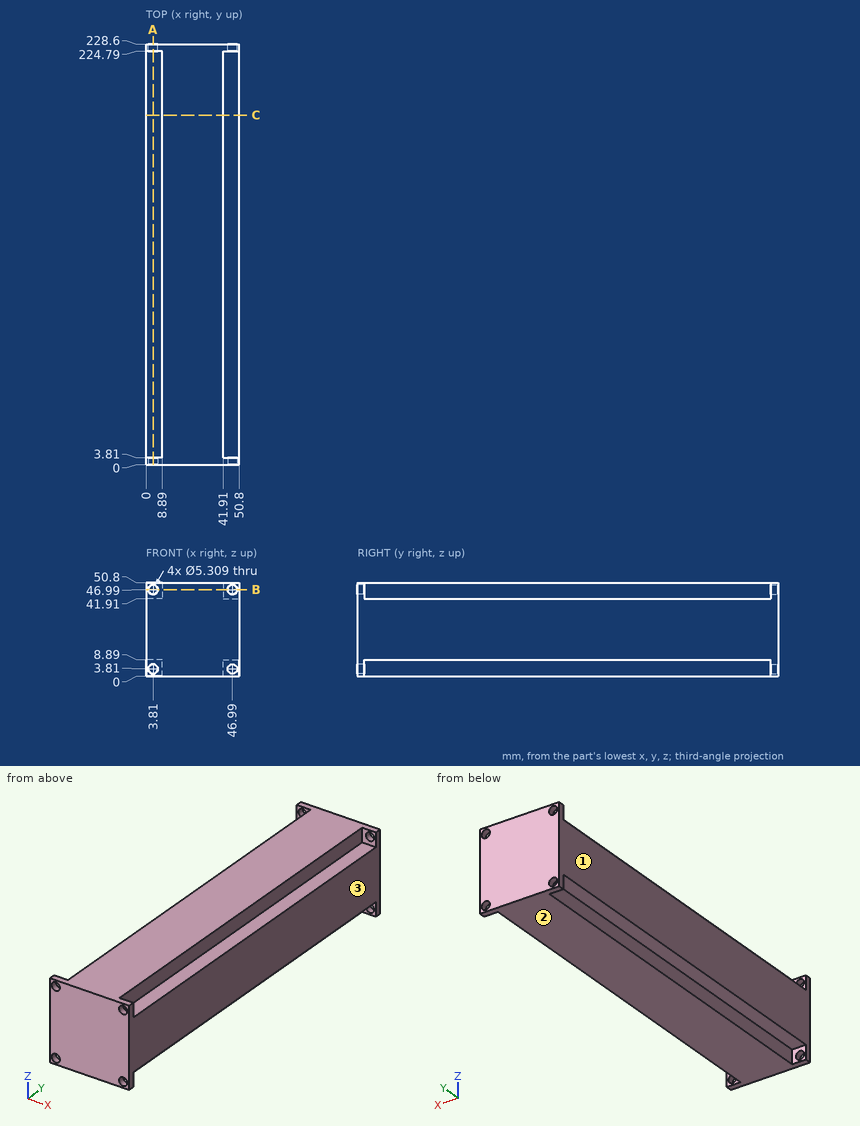
For this review, use the dimensioned drawing (mm, ordinates from the lowest corner) and the shaded views. Give positions to 0.01 mm unless a question says otherwise; leave off trailing zeros. Write each loop counter-clockwise with the first axis right and the second up, starting at its lowest first coordinate (ties: lowest second). Pieces come first, ordered by that corner, then holes. Notation, with made-up numbers: M 10.5,-26 L 36.5,-26 A21 ccw 36.5,8 Z; hole C 89.25,14 d7. An arc over 180 degrees is marked long. Answer as a JSON object with one key per item and string values. Group by question number.
1) For line 1 along Z through (x, y) = (3.81, 1.15) (1 decimal); line 2 along Z through (x, y) = (46, 1), list the stretches that pass through material, from the lowest coordinate up.
2) We need section A-A (x = 3.81). Give the boundary of the cut face in (y, z) (1 decimal).
3) Clearance check with flat-ended pins moving along their axes: pin 1 Ø7 at (x, z) = (47.5, 4.5) entering from -Y; pin 2 Ø4.5 at (y, z) = (122.5, 47.5) entering from +X; pin 3 Ø10 at (y, z) = (95.5, 47.5) entering from -X. State where each tip first meets the part, or that it passes through.
4) We need section C-C (y = 190). Give the boundary of the cut face in (x, z), and give its area (3 significant figures).
5) Mouldability with a two-part tool opening along X and no side actions: class the marked faces 1, 2 and 3 as released by +X, released by -X, zero draft, split by the parting line, or undercut.
6) We need section B-B (z = 46.99). Give the boundary of the cut face in (x, y) (1 decimal).
Answer key:
{
 "1": {"line 1": "z = 0 to 1.2, 6.5 to 44.3, 49.6 to 50.8", "line 2": "z = 0 to 1.35, 6.27 to 44.53, 49.45 to 50.8"},
 "2": {"outline": "M 0,0 L 3.8,0 L 3.8,1.2 L 0,1.2 Z; M 0,6.5 L 3.8,6.5 L 3.8,8.9 L 224.8,8.9 L 224.8,6.5 L 228.6,6.5 L 228.6,44.3 L 224.8,44.3 L 224.8,41.9 L 3.8,41.9 L 3.8,44.3 L 0,44.3 Z; M 0,49.6 L 3.8,49.6 L 3.8,50.8 L 0,50.8 Z; M 224.8,0 L 228.6,0 L 228.6,1.2 L 224.8,1.2 Z; M 224.8,49.6 L 228.6,49.6 L 228.6,50.8 L 224.8,50.8 Z"},
 "3": {"pin 1": "stops at y = 0", "pin 2": "stops at x = 41.91", "pin 3": "stops at x = 8.89"},
 "4": {"outline": "M 0,8.89 L 8.89,8.89 L 8.89,0 L 41.91,0 L 41.91,8.89 L 50.8,8.89 L 50.8,41.91 L 41.91,41.91 L 41.91,50.8 L 8.89,50.8 L 8.89,41.91 L 0,41.91 Z", "area": "2,260 mm²"},
 "5": {"face 1": "released by -X", "face 2": "zero draft", "face 3": "released by +X"},
 "6": {"outline": "M 0,0 L 1.2,0 L 1.2,3.8 L 0,3.8 Z; M 0,224.8 L 1.2,224.8 L 1.2,228.6 L 0,228.6 Z; M 6.5,0 L 44.3,0 L 44.3,3.8 L 41.9,3.8 L 41.9,224.8 L 44.3,224.8 L 44.3,228.6 L 6.5,228.6 L 6.5,224.8 L 8.9,224.8 L 8.9,3.8 L 6.5,3.8 Z; M 49.6,0 L 50.8,0 L 50.8,3.8 L 49.6,3.8 Z; M 49.6,224.8 L 50.8,224.8 L 50.8,228.6 L 49.6,228.6 Z"}
}
